```python
from build123d import *

# Parameters (mm, degrees)
SKETCH2_W           = 67.25
SKETCH2_H           = 42.5
BOSS_EXTRUDE1_DEPTH = 1.65
SKETCH3_R           = 1.7
CUT_EXTRUDE1_DEPTH  = 1.65
SKETCH5_R           = 0.5
CUT_EXTRUDE2_DEPTH  = 1.65
SKETCH8_R           = 0.5
CUT_EXTRUDE3_DEPTH  = 1.65


with BuildPart() as part:
    # Sketch2 → Boss-Extrude1 (new body)
    with BuildSketch(Plane.XY):
        Rectangle(SKETCH2_W, SKETCH2_H)
    extrude(amount=BOSS_EXTRUDE1_DEPTH)

    # Sketch3 → Cut-Extrude1 (cut)
    with BuildSketch(Plane(origin=(0, 0, 0), x_dir=(-1, 0, 0), z_dir=(0, 0, -1))):
        with Locations((31.125, -17.75)):
            Circle(SKETCH3_R)
        with Locations((31.125, 17.75)):
            Circle(SKETCH3_R)
        with Locations((-31.125, -17.75)):
            Circle(SKETCH3_R)
        with Locations((-31.125, 17.75)):
            Circle(SKETCH3_R)
    extrude(amount=-CUT_EXTRUDE1_DEPTH, mode=Mode.SUBTRACT)

    # Sketch5 → Cut-Extrude2 (cut)
    with BuildSketch(Plane.XY.offset(1.65)):
        with Locations((-31.125, 0)):
            Circle(SKETCH5_R)
        with Locations((-31.125, -2.54)):
            Circle(SKETCH5_R)
        with Locations((-31.125, -5.08)):
            Circle(SKETCH5_R)
        with Locations((-31.125, -7.62)):
            Circle(SKETCH5_R)
        with Locations((-31.125, -10.16)):
            Circle(SKETCH5_R)
        with Locations((-31.125, -12.7)):
            Circle(SKETCH5_R)
        with Locations((-31.125, 2.54)):
            Circle(SKETCH5_R)
        with Locations((-31.125, 5.08)):
            Circle(SKETCH5_R)
        with Locations((-31.125, 7.62)):
            Circle(SKETCH5_R)
        with Locations((-31.125, 10.16)):
            Circle(SKETCH5_R)
        with Locations((-31.125, 12.7)):
            Circle(SKETCH5_R)
    extrude(amount=-CUT_EXTRUDE2_DEPTH, mode=Mode.SUBTRACT)

    # Sketch8 → Cut-Extrude3 (cut)
    with BuildSketch(Plane.XY.offset(1.65)):
        with Locations((31.125, 0)):
            Circle(SKETCH8_R)
        with Locations((31.125, 2.54)):
            Circle(SKETCH8_R)
        with Locations((31.125, 5.08)):
            Circle(SKETCH8_R)
        with Locations((31.125, -2.54)):
            Circle(SKETCH8_R)
        with Locations((31.125, -5.08)):
            Circle(SKETCH8_R)
    extrude(amount=-CUT_EXTRUDE3_DEPTH, mode=Mode.SUBTRACT)


solid = part.part
```
Source: CAD feature listing. Evaluate the final solid. Frame: model axes, mm. Give positions to 0.01 mm unless a question says otherwise; leave off trailing zeros. Loops run counter-clockwise (first coordinate to the right, second up) from the corner with the lowest first, then second, coordinate; pieces in that order, holes last. Notation, with made-up numbers: (20, -14) -> (59, -14) arc R31 ccw to (59, 20) -> close; hole circle Ø2 at (-7.75, 25.5). An arc over 180 degrees is marked (long way). Use a Markdown table: item, result. Add a question column.
(1) Pull-direction query (X, two-part tool) for faces 1 (the face through (29.555, 17.099, 0.813)), 2 (the face through (0, -21.25, 1)), 3 (the face through (33.625, 0, 1)), 4 (the face through (-33.625, 0, 1)); classes: +X half, -X half, draft (parallel to the pull), parting line (faces both ways), or undercut.
(2) Section query A-A (z = 0.4). Count the separate pieces of the cut face and the enclosed holes in it, then the cut area to 3 significant figures.
(3) Section query B-B (y = 17.75). Output: boundary loops of the cut face in (x, z) (3 decimals), then the cut area to 3 significant figures.
(4) Ray query, line 1 (X direction, y = 19, z = 0.7) (3 decimals); line 2 (Y direction, x = 30, z = 0.15); line 3 (X direction, y = -10, z = 0.8) (3 decimals). Return the intervals inside material, ascending.
Checked values:
| question | item | result |
|---|---|---|
| 1 | face 1 | undercut |
| 1 | face 2 | draft |
| 1 | face 3 | +X half |
| 1 | face 4 | -X half |
| 2 | separate pieces | 1 |
| 2 | enclosed holes | 20 |
| 2 | area | 2,810 mm^2 |
| 3 | outline | (-33.625, 0) -> (-32.825, 0) -> (-32.825, 1.65) -> (-33.625, 1.65) -> close; (-29.425, 0) -> (29.425, 0) -> (29.425, 1.65) -> (-29.425, 1.65) -> close; (32.825, 0) -> (33.625, 0) -> (33.625, 1.65) -> (32.825, 1.65) -> close |
| 3 | area | 99.7 mm^2 |
| 4 | line 1 | -33.625 to -32.277, -29.973 to 29.973, 32.277 to 33.625 |
| 4 | line 2 | -21.25 to -19.02, -16.48 to 16.48, 19.02 to 21.25 |
| 4 | line 3 | -33.625 to -31.599, -30.651 to 33.625 |
